Autodesk Inventor part; units mm, degrees
ref_plane "YZ Plane" through (0, 0, 0) normal (1, 0, 0) x (0, 1, 0)
ref_plane "XZ Plane" through (0, 0, 0) normal (0, 1, 0) x (-1, 0, 0)
ref_plane "XY Plane" through (0, 0, 0) normal (0, 0, 1) x (1, 0, 0)
sketch "Skizze1" plane through (0, 0, 0) normal (0, 0, 1) x (1, 0, 0)
  line L0 (71.8801, -4.4448) -> (67.8801, -4.4448)
  line L1 (67.8801, -4.4448) -> (67.8801, -55.4448)
  line L2 (67.8801, -55.4448) -> (71.8801, -55.4448)
  line L3 (71.8801, -55.4448) -> (71.8801, -4.4448)
  line L4 (67.8801, -55.4448) -> (41.8801, -55.4448)
  line L5 (41.8801, -55.4448) -> (41.8801, -4.4448)
  line L6 (41.8801, -4.4448) -> (67.8801, -4.4448)
  line L7 (67.8801, -4.4448) -> (67.8801, -55.4448)
  line L8 (41.8801, -55.4448) -> (37.8801, -55.4448)
  line L9 (37.8801, -55.4448) -> (37.8801, -4.4448)
  line L10 (37.8801, -4.4448) -> (41.8801, -4.4448)
  line L11 (41.8801, -4.4448) -> (41.8801, -55.4448)
  point P0 (0, 0)
  dimension "d0" = 4
  dimension "d1" = 51
  dimension "d2" = 26
  dimension "d3" = 4
extrude "Extrusion1" add sketch "Skizze1" along normal blind 3.5 contours L3 L2 L1 L0 | L5 L8 L9 L10
sketch "Skizze2" plane through (0, 0, 3.5) normal (0, 0, 1) x (1, 0, 0)
  line L0 (71.8801, -55.4448) -> (37.8801, -55.4448)
  line L1 (71.8801, -4.4448) -> (37.8801, -4.4448)
  line L2 (37.8801, -4.4448) -> (37.8801, -55.4448)
  line L3 (71.8801, -55.4448) -> (71.8801, -4.4448)
  line L4 (43.3801, -4.4448) -> (66.3801, -4.4448)
  line L5 (66.3801, -4.4448) -> (66.3801, -21.4448)
  line L6 (66.3801, -21.4448) -> (43.3801, -21.4448)
  line L7 (43.3801, -21.4448) -> (43.3801, -4.4448)
  line L8 (41.8801, -55.4448) -> (67.8801, -55.4448)
  line L9 (59.8801, -55.4448) -> (59.8801, -25.4448)
  line L10 (59.8801, -25.4448) -> (49.8801, -25.4448)
  line L11 (49.8801, -25.4448) -> (49.8801, -55.4448)
  line L12 (41.8801, -55.4448) -> (67.8801, -55.4448)
  line L13 (67.8801, -55.4448) -> (67.8801, -55.4448)
  line L14 (67.8801, -55.4448) -> (41.8801, -55.4448)
  line L15 (41.8801, -55.4448) -> (41.8801, -55.4448)
  line L16 (54.8801, -55.4448) -> (54.8801, -25.4448) construction
  point P0 (0, 0)
  point P1 (54.8801, -4.4448)
  point P2 (67.8801, -45.4448)
  dimension "d38" = 23
  dimension "d39" = 17
  dimension "d44" = 4
  dimension "d47" = 26
  dimension "d54" = 10
extrude "Extrusion2" add sketch "Skizze2" along normal blind 2 contours L0 L9 L10 L11 L2 L1 L7 L6 L5 L3
sketch "Skizze3" plane through (0, 0, 5.5) normal (0, 0, 1) x (1, 0, 0)
  line L0 (37.8801, -4.4448) -> (37.8801, -55.4448)
  line L1 (39.8801, -23.4448) -> (37.8801, -23.4448) construction
  line L2 (39.8801, -23.4448) -> (41.8801, -23.4448) construction
  line L3 (39.8801, -23.4448) -> (39.8801, -4.4448) construction
  line L4 (69.8801, -23.4448) -> (71.8801, -23.4448) construction
  line L5 (71.8801, -4.4448) -> (37.8801, -4.4448) construction
  line L6 (71.8801, -55.4448) -> (71.8801, -4.4448)
  line L7 (71.8801, -55.4448) -> (37.8801, -55.4448)
  line L8 (37.8801, -55.4448) -> (71.8801, -55.4448)
  line L9 (39.8801, -53.4448) -> (39.8801, -23.4448)
  line L10 (69.8801, -53.4448) -> (69.8801, -23.4448)
  line L11 (67.8801, -4.4448) -> (67.8801, -55.4448)
  line L12 (39.8801, -53.4448) -> (39.8801, -55.4448)
  line L13 (69.8801, -53.4448) -> (69.8801, -55.4448)
  point P0 (0, 0)
  dimension "d24" = 2
  dimension "d37" = 19
hole "Bohrung1" at (39.8801, -23.4448, 5.5) at (69.8801, -23.4448, 5.5) at (39.8801, -53.4448, 5.5) at (69.8801, -53.4448, 5.5) direction (0, 0, -1) diameter 2.2 end through all countersink diameter 5 countersink angle 90
sketch "Skizze6" plane through (0, 0, 3.5) normal (0, 0, -1) x (-1, 0, 0)
  line L0 (-67.8801, -4.4448) -> (-67.8801, -55.4448)
  line L1 (-66.3801, -4.4448) -> (-66.3801, -21.4448)
  line L2 (-67.8801, -4.4448) -> (-66.3801, -4.4448)
  line L3 (-66.3801, -4.4448) -> (-66.3801, -10.4448)
  line L4 (-66.3801, -10.4448) -> (-67.8801, -10.4448)
  line L5 (-67.8801, -10.4448) -> (-67.8801, -4.4448)
  line L6 (-43.3801, -21.4448) -> (-43.3801, -4.4448)
  line L7 (-41.8801, -55.4448) -> (-41.8801, -4.4448)
  line L8 (-43.3801, -4.4448) -> (-41.8801, -4.4448)
  line L9 (-41.8801, -4.4448) -> (-41.8801, -10.4448)
  line L10 (-41.8801, -10.4448) -> (-43.3801, -10.4448)
  line L11 (-43.3801, -10.4448) -> (-43.3801, -4.4448)
  line L12 (-41.8801, -55.4448) -> (-49.8801, -55.4448)
  line L13 (-49.8801, -55.4448) -> (-49.8801, -52.4448)
  line L14 (-49.8801, -52.4448) -> (-41.8801, -52.4448)
  line L15 (-41.8801, -52.4448) -> (-41.8801, -55.4448)
  line L16 (-59.8801, -52.4448) -> (-59.8801, -55.4448)
  line L17 (-67.8801, -55.4448) -> (-59.8801, -55.4448)
  line L18 (-59.8801, -55.4448) -> (-59.8801, -52.4448)
  line L19 (-59.8801, -52.4448) -> (-67.8801, -52.4448)
  line L20 (-67.8801, -52.4448) -> (-67.8801, -55.4448)
  point P0 (0, 0)
  dimension "d48" = 6
extrude "Extrusion5" add sketch "Skizze6" along normal up to surface (3.5 mm away) contours L2 L1 L4 L0 | L6 L8 L7 L10
extrude "Extrusion6" add sketch "Skizze6" along normal blind 4 contours L19 L16 L17 L0 | L7 L12 L13 L14
properties part number "Sliderhalter" material "PC/ABS-Kunststoff, 3DDruck, PLA"
The model under review builds one solid part; all positions refer to its coordinate system, in mm. A direction names the side the tool comes from. Round coordinates to 2 decimals unless told otherwise and drop trailing zeros. Loops run counter-clockwise (first coordinate to the right, second up) from the corner with the lowest first, then second, coordinate; pieces in that order, holes last.
Item 1: Take a section at C-C (x = 60.5). Write out the cut boundary in (y, z).
Determined:
outline: (-55.44, -0.5) - (-52.44, -0.5) - (-52.44, 3.5) - (-21.44, 3.5) - (-21.44, 5.5) - (-55.44, 5.5) - close
Item 2: Take a section at D-D (y = -29). Write out the cut boundary in (x, z), then the cut area to 3 significant figures.
Determined:
outline: (37.88, 0) - (41.88, 0) - (41.88, 3.5) - (49.88, 3.5) - (49.88, 5.5) - (37.88, 5.5) - close; (59.88, 3.5) - (67.88, 3.5) - (67.88, 0) - (71.88, 0) - (71.88, 5.5) - (59.88, 5.5) - close
area: 76.0 mm2
Item 3: Take a section at B-B (z = 2.35). Write out the cut boundary in (x, y), then the cut area to 3 significant figures.
Determined:
outline: (37.88, -55.44) - (49.88, -55.44) - (49.88, -52.44) - (41.88, -52.44) - (41.88, -10.44) - (43.38, -10.44) - (43.38, -4.44) - (37.88, -4.44) - close; (59.88, -55.44) - (71.88, -55.44) - (71.88, -4.44) - (66.38, -4.44) - (66.38, -10.44) - (67.88, -10.44) - (67.88, -52.44) - (59.88, -52.44) - close; hole circle Ø2.2 at (39.88, -53.44); hole circle Ø2.2 at (39.88, -23.44); hole circle Ø2.2 at (69.88, -53.44); hole circle Ø2.2 at (69.88, -23.44)
area: 459 mm2
Item 4: Clearance check with flat-ended pins moving along their axes: pin 1 Ø3 at (x, y) = (41.5, -27.5) entering from -Z; pin 2 Ø2 at (x, z) = (66, 4) entering from +Y; pin 3 Ø0.6 at (x, z) = (57.5, 5) entering from +Y; pin 4 Ø1 at (x, z) = (56, 4) entering from -Y. State where each tip first meets the part, or that it passes through.
Determined:
pin 1: stops at z = 0
pin 2: stops at y = -4.44
pin 3: stops at y = -21.44
pin 4: stops at y = -25.44
Item 5: For faces 1 (the face through (43.38, -11, 4)), 2 (the face through (40.788, -52.455, 4.343)), 3 (the face through (64, -52.445, 2)), 4 (the face through (59.88, -44, 4)), list the 3-axis set-ups (+Z, -Z, +X, -X, +Y, -Y) from which the entire face can be reached by the end or side of a thin tool; tool diameter is ignored.
Determined:
face 1: +Z, -Z, +Y
face 2: +Z
face 3: -Z
face 4: +Z, -Z, -Y
Item 6: For line 1 (X direction, y = -32, z = 3.25); line 2 (X direction, y = -9, z = 0.1); line 3 (Y direction, x = 66.5, z = 3.25), list the stretches that pass through material, from the lowest coordinate up.
Determined:
line 1: x = 37.88 to 41.88, 67.88 to 71.88
line 2: x = 37.88 to 43.38, 66.38 to 71.88
line 3: y = -55.44 to -52.44, -10.44 to -4.44
Item 7: Take a section at A-A (y = -17). Write out the cut boundary in (x, z), then the cut area to 3 significant figures.
Determined:
outline: (37.88, 0) - (41.88, 0) - (41.88, 3.5) - (43.38, 3.5) - (43.38, 5.5) - (37.88, 5.5) - close; (66.38, 3.5) - (67.88, 3.5) - (67.88, 0) - (71.88, 0) - (71.88, 5.5) - (66.38, 5.5) - close
area: 50.0 mm2
Item 8: Mouldability with a two-part tool opening along Y and no side actions: class faces 5 (the face through (41, -4.445, 3)), 6 (the face through (37.88, -30, 3)), 7 (the face through (40.3, -54.46, 2.02)), 8 (the face through (44, -55.445, 2)) as released by +Y, released by -Y, zero draft, split by the parting line, or undercut.
Determined:
face 5: released by +Y
face 6: zero draft
face 7: undercut
face 8: released by -Y
